```python
from build123d import *

# Parameters (mm, degrees)
SKETCH1_W           = 19.05
SKETCH1_H           = 36.703
BOSS_EXTRUDE1_DEPTH = 22.4028
BOSS_EXTRUDE2_DEPTH = 7.62
SKETCH3_R           = 1.4859
CUT_EXTRUDE1_DEPTH  = 20.05
FILLET1_R           = 3.81
SKETCH6_W           = 2.921
SKETCH6_H           = 5.0292
BOSS_EXTRUDE3_DEPTH = 4.8006
FILLET2_R           = 0.254
SKETCH7_R           = 1.4097
CUT_EXTRUDE2_DEPTH  = 11.4521
BOSS_EXTRUDE4_DEPTH = 26.1112
SKETCH11_W          = 3.2004
SKETCH11_H          = 5.1562
BOSS_EXTRUDE5_DEPTH = 2.54
SKETCH12_W          = 8.4582
SKETCH12_H          = 7.62
BOSS_EXTRUDE6_DEPTH = 1.4224
BOSS_EXTRUDE7_DEPTH = 1.3843
SKETCH14_R          = 0.9906
BOSS_EXTRUDE8_DEPTH = 1.016


with BuildPart() as part:
    # Sketch1 → Boss-Extrude1 (new body)
    with BuildSketch(Plane(origin=(0, 0, 0), x_dir=(1, 0, 0), z_dir=(0, 1, 0))):
        Rectangle(SKETCH1_W, SKETCH1_H)
    extrude(amount=BOSS_EXTRUDE1_DEPTH)

    # Sketch2 → Boss-Extrude2 (add)
    with BuildSketch(Plane(origin=(9.525, 0, 0), x_dir=(0, 0, -1), z_dir=(1, 0, 0))):
        with BuildLine():
            Line((9.297778198, 14.092814896), (4.98725526, 14.092814896))
            ThreePointArc((4.98725526, 14.092814896), (4.348516729, 12.314814896), (4.98725526, 10.536814896))
            Line((4.98725526, 10.536814896), (9.297778198, 10.536814896))
            ThreePointArc((9.297778198, 10.536814896), (9.771987831, 11.370189188), (9.936516729, 12.314814896))
            ThreePointArc((9.936516729, 12.314814896), (9.771987831, 13.259440604), (9.297778198, 14.092814896))
        make_face()
    extrude(amount=BOSS_EXTRUDE2_DEPTH)

    # Sketch3 → Cut-Extrude1 (cut, through all)
    with BuildSketch(Plane(origin=(9.525, 0, 0), x_dir=(0, 0, -1), z_dir=(1, 0, 0))):
        with Locations((-12.8905, 19.9517)):
            Circle(SKETCH3_R)
        with Locations((-12.8905, 2.4511)):
            Circle(SKETCH3_R)
    extrude(amount=-CUT_EXTRUDE1_DEPTH, mode=Mode.SUBTRACT)

    # Fillet1
    fillet1_edges = [part.edges().sort_by_distance(p)[0] for p in [
        (0, 22.4028, -18.3515),
        (0, 0, -18.3515),
    ]]
    fillet(fillet1_edges, radius=FILLET1_R)

    # Sketch6 → Boss-Extrude3 (add)
    with BuildSketch(Plane(origin=(0, 0, -18.3515), x_dir=(-1, 0, 0), z_dir=(0, 0, -1))):
        with Locations((0.5334, 11.2014)):
            Rectangle(SKETCH6_W, SKETCH6_H)
    extrude(amount=BOSS_EXTRUDE3_DEPTH)

    # Fillet2
    fillet2_edges = [part.edges().sort_by_distance(p)[0] for p in [
        (-0.5334, 8.6868, -18.3515),
        (-0.5334, 13.716, -18.3515),
        (-0.5334, 8.6868, -23.1521),
        (-0.5334, 13.716, -23.1521),
    ]]
    fillet(fillet2_edges, radius=FILLET2_R)

    # Sketch7 → Cut-Extrude2 (cut, through all)
    with BuildSketch(Plane(origin=(0.9271, 0, 0), x_dir=(0, 0, -1), z_dir=(1, 0, 0))):
        with Locations((20.7518, 11.2014)):
            Circle(SKETCH7_R)
    extrude(amount=-CUT_EXTRUDE2_DEPTH, mode=Mode.SUBTRACT)

    # Sketch8 → Boss-Extrude4 (add)
    with BuildSketch(Plane.XY.offset(18.3515)):
        with BuildLine():
            Line((-9.525, 17.9451), (-9.525, 4.4577))
            ThreePointArc((-9.525, 4.4577), (-0.724870396, -0.036468986), (8.22325, 4.155305974))
            Line((8.22325, 4.155305974), (8.22325, 18.247494026))
            ThreePointArc((8.22325, 18.247494026), (-0.724870396, 22.439268986), (-9.525, 17.9451))
        make_face()
    extrude(amount=BOSS_EXTRUDE4_DEPTH)

    # Sketch11 → Boss-Extrude5 (add)
    with BuildSketch(Plane.ZY.offset(9.525)):
        with Locations((24.4729, 11.2014)):
            Rectangle(SKETCH11_W, SKETCH11_H)
    boss_extrude5 = extrude(amount=BOSS_EXTRUDE5_DEPTH)

    # Mirror1: Boss-Extrude5 across plane
    add(boss_extrude5.mirror(Plane(origin=(-0.650875, 0, 0), x_dir=(0, 0, 1), z_dir=(1, 0, 0))))

    # Sketch12 → Boss-Extrude6 (add)
    with BuildSketch(Plane.ZY.offset(9.525)):
        with Locations((40.2336, 11.2014)):
            Rectangle(SKETCH12_W, SKETCH12_H)
    extrude(amount=BOSS_EXTRUDE6_DEPTH)

    # Sketch13 → Boss-Extrude7 (add)
    with BuildSketch(Plane.XY.offset(44.4627)):
        with BuildLine():
            Line((3.159125, 8.076477319), (3.159125, 14.326322681))
            ThreePointArc((3.159125, 14.326322681), (-5.578475, 11.2014), (3.159125, 8.076477319))
        make_face()
    extrude(amount=BOSS_EXTRUDE7_DEPTH)

    # Sketch14 → Boss-Extrude8 (add)
    with BuildSketch(Plane.XY.offset(45.847)):
        with Locations((-0.650875, 11.2014)):
            Circle(SKETCH14_R)
    extrude(amount=BOSS_EXTRUDE8_DEPTH)


solid = part.part
```
Geometry: final body of the model. Coordinates: model frame, mm. A direction names the side the tool comes from. Round coordinates to 2 decimals unless told otherwise and drop trailing zeros. Write each loop counter-clockwise with the first axis right and the second up, starting at its lowest first coordinate (ties: lowest second). Pieces come first, ordered by that corner, then holes.
Item 1: Mould query, pull axis Z, two halves, no side actions, for faces 5 (the face through (9, 11, 26.073)), 6 (the face through (-1, 8.687, -21)), 7 (the face through (0.13, 1.09, -17.21)), 8 (the face through (-0.513, 11.263, -19.343)). Classes: +Z half, -Z half, draft (parallel to the pull), parting line (faces both ways), or undercut.
Item 2: Section query C-C (z = 30). Return loops of the section in (x, y) (1 decimal).
Item 3: Set-up query: faces 1 (the face through (-10.947, 11, 40)), 2 (the face through (9, 13.779, 24)), 3 (the face through (-11, 8.623, 24)), 4 (the face through (13, 10.537, -7)). Return all of +Z, -Z, +X, -X, +Y, -Y with unobstructed straight access to the full face (end or side cutting, diameter ignored); none if empty.
Item 4: Material intervals for L1, parallel to Z at x = 3.75, y = 7.5; L2, parallel to X at y = 15.75, z = -13.5 (3 decimals); L3, parallel to Y at x = 1.75, z = -2, sorted ascending.
Item 5: Section query B-B (x = 13.25). Return loops of the section in (y, z), plus the area to 3 significant figures.
Item 6: Section query D-D (x = 5.5). Return loops of the section in (y, z).
Item 7: Pin query (flat end, axial travel): P1, Ø8, axis at x = 8.5, z = -6.5, coming from the -Y side; P2, Ø12, axis at x = 1.5, y = 9.5, coming from the +Z side; P3, Ø8, axis at x = 12, y = 20, coming from the -Z side; P4, Ø2.5, axis at y = 12, z = -20, coming from the -X side. Return the tip coordinate at first contact, or that it passes through.
Item 8: Section query A-A (x = -6.25). Return loops of the section in (y, z).
Completed:
1. face 5: +Z half
1. face 6: draft
1. face 7: -Z half
1. face 8: undercut
2. outline: (-9.5, 4.5) arc R11.2 ccw to (8.2, 4.2) - (8.2, 18.2) arc R11.2 ccw to (-9.5, 17.9) - close
3. face 1: +Z, -X, +Y, -Y
3. face 2: +Z, +X, +Y
3. face 3: -Z, -X, -Y
3. face 4: -Z, +X, -Y
4. L1: z = -18.35 to 44.46
4. L2: x = -9.525 to 9.525
4. L3: y = 0 to 22.4
5. outline: (10.54, -9.3) arc R2.79 ccw to (14.09, -9.3) - (14.09, -4.99) arc R2.79 ccw to (10.54, -4.99) - close
5. area: 18.4 mm2
6. outline: (0, -14.54) arc R3.81 ccw to (3.81, -18.35) - (18.59, -18.35) arc R3.81 ccw to (22.4, -14.54) - (22.4, 18.35) - (20.68, 18.35) - (20.68, 44.46) - (1.72, 44.46) - (1.72, 18.35) - (0, 18.35) - close; hole circle Ø2.97 at (2.45, 12.89); hole circle Ø2.97 at (19.95, 12.89)
7. P1: stops at y = 0
7. P2: stops at z = 46.86
7. P3: stops at z = -18.35
7. P4: stops at x = -1.99
8. outline: (0, -14.54) arc R3.81 ccw to (3.81, -18.35) - (18.59, -18.35) arc R3.81 ccw to (22.4, -14.54) - (22.4, 18.35) - (20.88, 18.35) - (20.88, 44.46) - (1.52, 44.46) - (1.52, 18.35) - (0, 18.35) - close; hole circle Ø2.97 at (2.45, 12.89); hole circle Ø2.97 at (19.95, 12.89)
